The drawing under review shows one solid part. Ordinate dimensions are in mm from its lowest x, y, z. A direction names the side the tool comes from. Give positions to 0.01 mm unless a question says otherwise; leave off trailing zeros. Write each loop counter-clockwise with the first axis right and the second up, starting at its lowest first coordinate (ties: lowest second). Pieces come first, ordered by that corner, then holes. Notation, with made-up numbers: (68.25, -24.75) -> (78.25, -24.75) arc R12 ccw to (78.25, -12.75) -> close; hole circle Ø4 at (31, 50.5). An arc over 180 degrees is marked (long way). Answer as a JSON object with one key per item and string values.
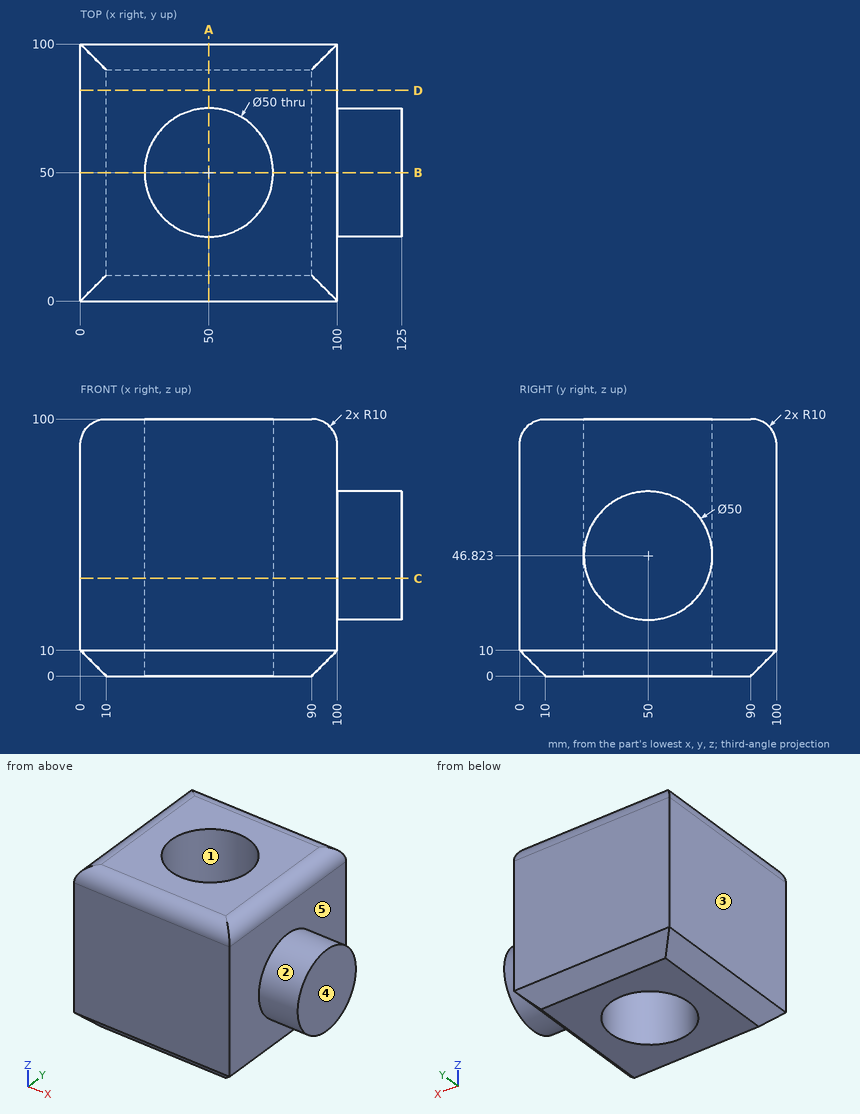
(1) For the marked faces 4 and 5, list the 3-axis set-ups (+Z, -Z, +X, -X, +Y, -Y) from which the entire face can be reached by the end or side of a thin tool; tool diameter is ignored.
Here are the results:
{"face 4": "+Z, -Z, +X, +Y, -Y", "face 5": "+X"}
(2) We need section B-B, the plane y = 50. State the section outline as (x, z) points, then the cut area to 3 significant figures.
Here are the results:
{"outline": "(0, 10) -> (10, 0) -> (25, 0) -> (25, 100) -> (10, 100) arc R10 ccw to (0, 90) -> close; (75, 0) -> (90, 0) -> (100, 10) -> (100, 21.82) -> (125, 21.82) -> (125, 71.82) -> (100, 71.82) -> (100, 90) arc R10 ccw to (90, 100) -> (75, 100) -> close", "area": "6,110 mm²"}
(3) We need section C-C, the plane z = 38. State the section outline as (x, y) points, then the cut area to 3 significant figures.
Here are the results:
{"outline": "(0, 0) -> (100, 0) -> (100, 26.61) -> (125, 26.61) -> (125, 73.39) -> (100, 73.39) -> (100, 100) -> (0, 100) -> close; hole circle Ø50 at (50, 50)", "area": "9,210 mm²"}
(4) Clearance check with a flat-ended pin moving along its axis: pin 1 (4 mm diameter, centred on y = 74.5, z = 65, fed in from +X). State where the tip first meets the part, or that it passes through.
Here are the results:
{"pin 1": "stops at x = 100"}
(5) We need section A-A, the plane x = 50. State the section outline as (y, z) points, then the cut area to 3 significant figures.
Here are the results:
{"outline": "(0, 10) -> (10, 0) -> (25, 0) -> (25, 100) -> (10, 100) arc R10 ccw to (0, 90) -> close; (75, 0) -> (90, 0) -> (100, 10) -> (100, 90) arc R10 ccw to (90, 100) -> (75, 100) -> close", "area": "4,860 mm²"}
(6) The part is to be moulded in two halves that separate along Y. For the marked faces 1, 2 and 3, say which applies: +Y half, -Y half, draft (parallel to the pull), parting line (faces both ways), or undercut.
Here are the results:
{"face 1": "undercut", "face 2": "parting line", "face 3": "draft"}
(7) We need section D-D, the plane y = 82. State the section outline as (x, z) points, then the cut area to 3 significant figures.
Here are the results:
{"outline": "(0, 10) -> (10, 0) -> (90, 0) -> (100, 10) -> (100, 90) arc R10 ccw to (90, 100) -> (10, 100) arc R10 ccw to (0, 90) -> close", "area": "9,860 mm²"}
(8) For line 1 along Y through (x, z) = (50, 57); line 2 along X through (y, z) = (62, 52.5); line 3 along X through (y, z) = (15, 36.5), list the stretches that pass through material, from the lowest coordinate up.
Here are the results:
{"line 1": "y = 0 to 25, 75 to 100", "line 2": "x = 0 to 28.07, 71.93 to 125", "line 3": "x = 0 to 100"}
